Can you work these out from the model? Positions are in its coordinate system, mm. Round coordinates to 2 decimals unless told otherwise and drop trailing zeros. Loops run counter-clockwise (first coordinate to the right, second up) from the corner with the lowest first, then second, coordinate; pieces in that order, holes last. Notation, with made-up numbers: M 45,-2.5 L 94,-2.5 A9 ccw 94,2.5 Z; hole C 71.25,-18.5 d8. An arc over 180 degrees is marked long. Return JSON: item names as keys, results as strings.
```python
from build123d import *

# Parameters (mm, degrees)
BOSS_EXTRUDE1_DEPTH = 3.6068
SKETCH2_W           = 4.5593
SKETCH2_H           = 2.032
HOLE1_D             = 6.4008
HOLE1_DEPTH         = 5.6388


with BuildPart() as part:
    # Sketch1 → Boss-Extrude1 (new body)
    with BuildSketch(Plane.XY.offset(1.8034)):
        with BuildLine():
            Line((9.576261807, 8.1026), (-9.576261807, 8.1026))
            ThreePointArc((-9.576261807, 8.1026), (-12.4968, 0), (-9.576261807, -8.1026))
            Line((-9.576261807, -8.1026), (9.576261807, -8.1026))
            ThreePointArc((9.576261807, -8.1026), (12.4968, 0), (9.576261807, 8.1026))
        make_face()
    extrude(amount=-BOSS_EXTRUDE1_DEPTH)

    # Sketch2 → Revolve1 (revolve)
    with BuildSketch(Plane(origin=(0, 0, 0), x_dir=(1, 0, 0), z_dir=(0, 1, 0))):
        with Locations((-3.07975, -2.8194)):
            Rectangle(SKETCH2_W, SKETCH2_H)
    revolve(axis=Axis((-5.3594, 0, 1.8034), (0, 0, 1)))

    # Hole1
    with Locations(Plane(origin=(0, 0, -1.8034), x_dir=(-1, 0, 0), z_dir=(0, 0, -1))):
        with Locations((5.3594, 0)):
            Hole(HOLE1_D / 2, depth=HOLE1_DEPTH)


solid = part.part
```
Q1. Suppose I cut it at B-B, the plane z = -1.05. Please give me the cut outline in (x, y).
Results:
{"outline": "M -9.58,-8.1 L 9.58,-8.1 A12.7 ccw 9.58,8.1 L -9.58,8.1 A12.7 ccw Z; hole C -5.36,0 d6.4"}
Q2. Suppose I cut it at D-D, the plane x = 1.5. Please give me the cut outline in (y, z).
Results:
{"outline": "M -8.1,-1.8 L 8.1,-1.8 L 8.1,1.8 L -8.1,1.8 Z"}
Q3. Suppose I cut it at A-A, the plane y = 0. Please give me the cut outline in (x, z), plus the area to 3 significant figures.
Results:
{"outline": "M -12.5,-1.8 L -8.56,-1.8 L -8.56,3.84 L -9.92,3.84 L -9.92,1.8 L -12.5,1.8 Z; M -2.16,-1.8 L 12.5,-1.8 L 12.5,1.8 L -0.8,1.8 L -0.8,3.84 L -2.16,3.84 Z", "area": "72.6 mm2"}
Q4. If I drill on line 1 along Y through (x, z) = (-5.5, 2.6); line 2 along Z through (x, y) = (5, -4.5); line 3 along Y through (x, z) = (-6.5, 3), over which ranges is the centre line in solid material (lowest first)?
Results:
{"line 1": "y = -4.56 to -3.2, 3.2 to 4.56", "line 2": "z = -1.8 to 1.8", "line 3": "y = -4.41 to -2.99, 2.99 to 4.41"}
Q5. Suppose I cut it at C-C, the plane y = 4.25. Please give me the cut outline in (x, z), plus the area to 3 significant figures.
Results:
{"outline": "M -11.76,-1.8 L 11.76,-1.8 L 11.76,1.8 L -3.71,1.8 L -3.71,3.84 L -7.01,3.84 L -7.01,1.8 L -11.76,1.8 Z", "area": "91.6 mm2"}
Q6. Thinking about a two-plate mould opening in X: for faces 1 (the cylindrical face through (-1.01, 1.37, 2.81)), 2 (the cylindrical face through (12.496, -0.123, 0.025)), 3 (the flat face through (0, 8.103, 0)), 4 (the cylindrical face through (-2.307, 0.961, 1.055)), which applies, pulls with the +X half, pulls with the -X half, needs draft (parallel to the pull), parting line crosses it, or undercut?
Results:
{"face 1": "parting line crosses it", "face 2": "pulls with the +X half", "face 3": "needs draft", "face 4": "undercut"}
Q7. I'm going to push flat-ended pins straight in: pin 1 Ø2 at (y, z) = (2, 0) entering from +X; pin 2 Ø3 at (y, z) = (6.5, 1) entering from +X; pin 3 Ø1.5 at (x, z) = (-8.5, 2.5) entering from +Y; pin 4 Ø4 at (x, y) = (4, 5) entering from +Z. Where does each tip first touch, or does it pass through?
Results:
{"pin 1": "stops at x = 12.46", "pin 2": "stops at x = 11.47", "pin 3": "stops at y = 8.1", "pin 4": "stops at z = 1.8"}
